```python
from build123d import *

# Parameters (mm, degrees)
AUFSATZ_LINEAR_AUSTRAGEN1_DEPTH = 65
SKIZZE3_R                       = 8
SCHNITT_LINEAR_AUSTRAGEN2_DEPTH = 85
SKIZZE4_W                       = 66
SKIZZE4_H                       = 25.15
SCHNITT_LINEAR_AUSTRAGEN3_DEPTH = 120
SKIZZE5_R                       = 2.5
SCHNITT_LINEAR_AUSTRAGEN4_DEPTH = 15
SKIZZE6_R                       = 2.5
SCHNITT_LINEAR_AUSTRAGEN5_DEPTH = 12
SKIZZE7_W                       = 21
SKIZZE7_H                       = 25.15
AUFSATZ_LINEAR_AUSTRAGEN2_DEPTH = 66
SKIZZE8_R                       = 2.5
SCHNITT_LINEAR_AUSTRAGEN7_DEPTH = 12
SCHNITT_LINEAR_AUSTRAGEN8_DEPTH = 5
SKIZZE10_W                      = 60
SKIZZE10_H                      = 10
AUFSATZ_LINEAR_AUSTRAGEN3_DEPTH = 2


with BuildPart() as part:
    # Skizze1 → Aufsatz-Linear austragen1 (new body)
    with BuildSketch(Plane.XY):
        Polygon((0, 0), (168, 0), (168, 10), (158, 10), (158, 50), (13, 50), (13, 10), (0, 10), align=None)
    extrude(amount=AUFSATZ_LINEAR_AUSTRAGEN1_DEPTH)

    # Skizze3 → Schnitt-Linear austragen2 (cut)
    with BuildSketch(Plane(origin=(0, 0, 0), x_dir=(-1, 0, 0), z_dir=(0, -1, 0))):
        with Locations((-108, -32.5)):
            Circle(SKIZZE3_R)
    extrude(amount=-SCHNITT_LINEAR_AUSTRAGEN2_DEPTH, mode=Mode.SUBTRACT)

    # Skizze4 → Schnitt-Linear austragen3 (cut)
    with BuildSketch(Plane(origin=(0, 0, 0), x_dir=(-1, 0, 0), z_dir=(0, 0, -1))):
        with Locations((-46, 37.425)):
            Rectangle(SKIZZE4_W, SKIZZE4_H)
    extrude(amount=-SCHNITT_LINEAR_AUSTRAGEN3_DEPTH, mode=Mode.SUBTRACT)

    # Skizze5 → Schnitt-Linear austragen4 (cut)
    with BuildSketch(Plane(origin=(158, 0, 0), x_dir=(0, 0, -1), z_dir=(1, 0, 0))):
        with Locations((-50, 40)):
            Circle(SKIZZE5_R)
        with Locations((-50, 22)):
            Circle(SKIZZE5_R)
        with Locations((-15, 22)):
            Circle(SKIZZE5_R)
        with Locations((-15, 40)):
            Circle(SKIZZE5_R)
    extrude(amount=-SCHNITT_LINEAR_AUSTRAGEN4_DEPTH, mode=Mode.SUBTRACT)

    # Skizze6 → Schnitt-Linear austragen5 (cut)
    with BuildSketch(Plane.ZY.offset(-13)):
        with Locations((15, 18)):
            Circle(SKIZZE6_R)
        with Locations((50, 18)):
            Circle(SKIZZE6_R)
    extrude(amount=-SCHNITT_LINEAR_AUSTRAGEN5_DEPTH, mode=Mode.SUBTRACT)

    # Skizze7 → Aufsatz-Linear austragen2 (add)
    with BuildSketch(Plane.ZY.offset(-13)):
        with Locations((10.5, 37.425)):
            Rectangle(SKIZZE7_W, SKIZZE7_H)
    extrude(amount=-AUFSATZ_LINEAR_AUSTRAGEN2_DEPTH)

    # Skizze8 → Schnitt-Linear austragen7 (cut)
    with BuildSketch(Plane.ZY.offset(-13)):
        with Locations((15, 40)):
            Circle(SKIZZE8_R)
    extrude(amount=-SCHNITT_LINEAR_AUSTRAGEN7_DEPTH, mode=Mode.SUBTRACT)

    # Skizze9 → Schnitt-Linear austragen8 (cut)
    with BuildSketch(Plane(origin=(0, 0, 0), x_dir=(-1, 0, 0), z_dir=(0, 0, -1))):
        Polygon((0, 0), (0, 10), (-13, 10), (-13, 50), (-158, 50), (-158, 10), (-168, 10), (-168, 0), align=None)
    extrude(amount=-SCHNITT_LINEAR_AUSTRAGEN8_DEPTH, mode=Mode.SUBTRACT)

    # Skizze10 → Aufsatz-Linear austragen3 (add)
    with BuildSketch(Plane.ZY):
        with Locations((35, 5)):
            Rectangle(SKIZZE10_W, SKIZZE10_H)
    extrude(amount=AUFSATZ_LINEAR_AUSTRAGEN3_DEPTH)


solid = part.part
```
Here's how the part is built. I have some questions about the finished solid (model axes, mm). A direction names the side the tool comes from. Coordinates: 2 decimals unless noted, no trailing zeros. Order: outer loops, then holes, each group sorted by start corner. A loop starts at its lowest first (then second) coordinate and runs counter-clockwise, first axis right, second up.
Item 1: If we section it at B-B, the plane x = 145: List the corners of the cut face in (y, z) for me.
Response values:
outline: (0, 5) - (50, 5) - (50, 65) - (0, 65) - close; hole circle Ø5 at (22, 15); hole circle Ø5 at (22, 50); hole circle Ø5 at (40, 15); hole circle Ø5 at (40, 50)
Item 2: If we section it at C-C, the plane z = 32.5: List the corners of the cut face in (x, y) for me, then the cut area to 3 significant figures.
Response values:
outline: (-2, 0) - (100, 0) - (100, 50) - (79, 50) - (79, 24.85) - (13, 24.85) - (13, 10) - (-2, 10) - close; (116, 0) - (168, 0) - (168, 10) - (158, 10) - (158, 50) - (116, 50) - close
area: 5,040 mm2
Item 3: If we section it at D-D, the plane z = 43.5: List the corners of the cut face in (x, y) for me, then the cut area to 3 significant figures.
Response values:
outline: (-2, 0) - (168, 0) - (168, 10) - (158, 10) - (158, 50) - (79, 50) - (79, 24.85) - (13, 24.85) - (13, 10) - (-2, 10) - close
area: 5,840 mm2
Item 4: If we section it at A-A, the plane y = 34: List the corners of the cut face in (x, z) for me.
Response values:
outline: (13, 5) - (158, 5) - (158, 65) - (79, 65) - (79, 21) - (13, 21) - close; hole circle Ø16 at (108, 32.5)
Item 5: I'm going to push flat-ended pins straight in: pin 1 Ø14.5 at (x, z) = (108, 32.5) entering from -Y; pin 2 Ø8 at (x, z) = (34.5, 43) entering from +Y; pin 3 Ø2.5 at (y, z) = (39, 49.5) entering from +X; pin 4 Ø4 at (y, z) = (17.5, 15.5) entering from -X. Where does each tip first touch, or does it pass through?
Response values:
pin 1: passes through
pin 2: stops at y = 24.85
pin 3: stops at x = 143
pin 4: stops at x = 13
Item 6: Which directions (+Z, -Z, +X, -X, +Y, -Y) give clear straight access to the entire face, cutting with the end or side of a thin tool? Please do faces 4 (the face through (150.6, 39.04, 47.69)), 5 (the face through (6, 10, 35)), 6 (the face through (46, 37, 21)), 7 (the face through (158, 30, 35)), 8 (the face through (18.92, 37.56, 14.46)).
Response values:
face 4: +X
face 5: +Z, -Z, -X, +Y
face 6: +Z, -X, +Y
face 7: +Z, -Z, +X, +Y
face 8: -X
Item 7: Thinking about a two-plate mould opening in Z: for faces 1 (the face through (168, 5, 35)), 2 (the face through (84, 25, 5)), 3 (the face through (150.6, 37.56, 15.54)), which applies, pulls with the +Z half, pulls with the -Z half, needs draft (parallel to the pull), parting line crosses it, or undercut?
Response values:
face 1: needs draft
face 2: pulls with the -Z half
face 3: undercut
Item 8: I need wall thicknesses on probe 1 along Y at (x, z) = (155, 50); probe 2 along Y at (x, z) = (16, 15); probe 3 along X at (y, z) = (16.5, 32.5). Which ranges of each line are inside material? Lowest first, please.
Response values:
probe 1: y = 0 to 19.5, 24.5 to 37.5, 42.5 to 50
probe 2: y = 0 to 15.5, 20.5 to 37.5, 42.5 to 50
probe 3: x = 13 to 100, 116 to 158
